Here's how the part is built. I have some questions about the finished solid (model axes, mm). Coordinates: 2 decimals unless noted, no trailing zeros. Order: outer loops, then holes, each group sorted by start corner. A loop starts at its lowest first (then second) coordinate and runs counter-clockwise, first axis right, second up. Notation, with made-up numbers: (31, 3) - (74, 3) arc R8 cw to (74, 8) - close; hole circle Ø2 at (78, -23.75). An arc over 180 degrees is marked (long way). Answer as CSV lines item,"result". Start each with the question number.
Item 1: I need wall thicknesses on line 1 (Z direction, x = 55, y = 5); line 2 (X direction, y = 5, z = 71); line 3 (Y direction, x = -45, z = 55). Which ranges of each line are inside material? Lowest first, please.
Item 2: Imagine slicing it at B-B on y = 118. List the corners of the cut face in (x, z) for me, and give its area (3 significant figures).
Item 3: I'm going to push flat-ended pins straight in: pin 1 (8.5 mm diameter, centred on x = 55, z = -71, fed in from -Y); pin 2 (4 mm diameter, centred on x = -67.5, z = 103, fed in from -Y); pin 3 (8 mm diameter, centred on x = -5.5, z = 32, fed in from +Y); pin 4 (11 mm diameter, centred on x = -55, z = -71, fed in from +Y). Where does each tip first touch, or does it pass through?
Item 4: Imagine slicing it at A-A on z = -57.5. List the corners of the cut face in (x, y) for me.
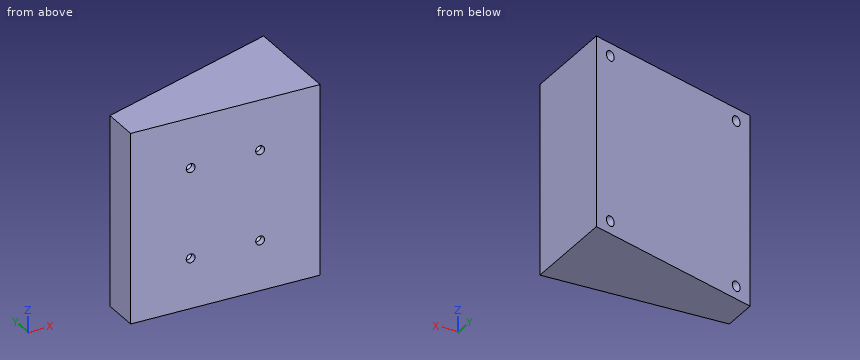
from build123d import *

# Parameters (mm, degrees)
ESBO_O1_W                            = 300
ESBO_O1_H                            = 300
RESSALTO_EXTRUS_O1_DEPTH             = 60
FURO_ROSCADO_DE_M16X2_01_D           = 14
FURO_ROSCADO_DE_M16X2_01_DEPTH       = 10
FURO_ROSCADO_DE_M16X2_01_TIP         = 4.206024333
RESSALTO_EXTRUS_O2_REACH             = 152
RESSALTO_EXTRUS_O2_DIRECTION_2_REACH = 152
FURO_ROSCADO_DE_M18X2_01_D           = 16
FURO_ROSCADO_DE_M18X2_01_DEPTH       = 18
FURO_ROSCADO_DE_M18X2_01_TIP         = 4.806884952


with BuildPart() as part:
    # Esboço1 → Ressalto-extrusão1 (new body)
    with BuildSketch(Plane(origin=(0, 0, 0), x_dir=(1, 0, 0), z_dir=(0, 1, 0))):
        Rectangle(ESBO_O1_W, ESBO_O1_H)
    extrude(amount=RESSALTO_EXTRUS_O1_DEPTH)

    # Furo roscado de M16x2.01
    with Locations(Plane(origin=(0, 0, 0), x_dir=(-1, 0, 0), z_dir=(0, -1, 0))):
        with Locations((55, -71), (-55, -71), (-55, 71), (55, 71)):
            Hole(FURO_ROSCADO_DE_M16X2_01_D / 2, depth=FURO_ROSCADO_DE_M16X2_01_DEPTH)
            with Locations((0, 0, -(FURO_ROSCADO_DE_M16X2_01_DEPTH + FURO_ROSCADO_DE_M16X2_01_TIP / 2))):  # 118° drill point
                Cone(0, FURO_ROSCADO_DE_M16X2_01_D / 2, FURO_ROSCADO_DE_M16X2_01_TIP, mode=Mode.SUBTRACT)

    # Ressalto-extrusão2: up to this face of the body (flat: up to its plane)
    ressalto_extrus_o2_end = Plane(part.part.faces().sort_by_distance((0, 30, 150))[0])
    # Esboço12 → Ressalto-extrusão2 (add, up to the picked face)
    with BuildSketch(Plane.XY, mode=Mode.PRIVATE) as ressalto_extrus_o2_sk1:
        Polygon((-150, 60), (150, 163.298283987), (150, 60), align=None)
    ressalto_extrus_o2_tool1 = split(extrude(ressalto_extrus_o2_sk1.sketch, amount=RESSALTO_EXTRUS_O2_REACH, mode=Mode.PRIVATE), bisect_by=ressalto_extrus_o2_end, keep=Keep.BOTH, mode=Mode.PRIVATE)
    add(ressalto_extrus_o2_tool1.solids().sort_by_distance((50, 94.432761, 0))[0])

    # Ressalto-extrusão2 direction 2: up to this face of the body (flat: up to its plane)
    ressalto_extrus_o2_direction_2_end = Plane(part.part.faces().sort_by_distance((0, 30, -150))[0])
    # Esboço12 → Ressalto-extrusão2 direction 2 (add, up to the picked face)
    with BuildSketch(Plane.XY, mode=Mode.PRIVATE) as ressalto_extrus_o2_direction_2_sk1:
        Polygon((-150, 60), (150, 163.298283987), (150, 60), align=None)
    ressalto_extrus_o2_direction_2_tool1 = split(extrude(ressalto_extrus_o2_direction_2_sk1.sketch, amount=-RESSALTO_EXTRUS_O2_DIRECTION_2_REACH, mode=Mode.PRIVATE), bisect_by=ressalto_extrus_o2_direction_2_end, keep=Keep.BOTH, mode=Mode.PRIVATE)
    add(ressalto_extrus_o2_direction_2_tool1.solids().sort_by_distance((50, 94.432761, 0))[0])

    # Furo roscado de M18x2.01
    with Locations(Plane(origin=(-34.369037739, 99.814933258, 0), x_dir=(0.945518576, 0.325568154, 0), z_dir=(-0.325568154, 0.945518576, 0))):
        with Locations((-93.650594894, 130), (166.349405106, 130), (166.349405106, -130), (-93.650594894, -130)):
            Hole(FURO_ROSCADO_DE_M18X2_01_D / 2, depth=FURO_ROSCADO_DE_M18X2_01_DEPTH)
            with Locations((0, 0, -(FURO_ROSCADO_DE_M18X2_01_DEPTH + FURO_ROSCADO_DE_M18X2_01_TIP / 2))):  # 118° drill point
                Cone(0, FURO_ROSCADO_DE_M18X2_01_D / 2, FURO_ROSCADO_DE_M18X2_01_TIP, mode=Mode.SUBTRACT)


solid = part.part
Responses:
1,line 1,"z = -150 to -78, -64 to 64, 78 to 150"
1,line 2,"x = -150 to -62, -48 to 48, 62 to 150"
1,line 3,"y = 0 to 96.15"
2,outline,"(18.44, -150) - (150, -150) - (150, 150) - (18.44, 150) - close"
2,area,"39,500 mm^2"
3,pin 1,"stops at y = 11.65"
3,pin 2,"stops at y = 0"
3,pin 3,"stops at y = 111.13"
3,pin 4,"stops at y = 94.6"
4,outline,"(-150, 0) - (150, 0) - (150, 163.3) - (-150, 60) - close"
